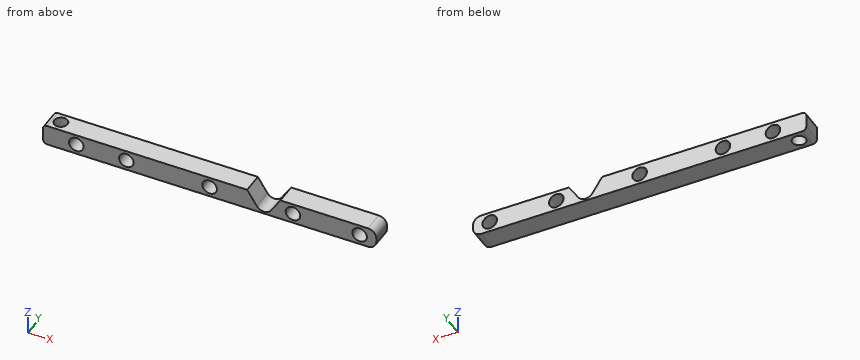
from build123d import *

# Parameters (mm, degrees)
SKETCH1_W           = 101.6
SKETCH1_H           = 6.35
BOSS_EXTRUDE1_DEPTH = 6.35
FILLET1_R           = 2.54
FILLET2_R           = 1.27
CUT_EXTRUDE1_REACH  = 53.294
SKETCH2_R           = 2.2225
CUT_EXTRUDE2_REACH  = 53.588
SKETCH3_R           = 2.032
CUT_EXTRUDE3_REACH  = 53.294


with BuildPart() as part:
    # Sketch1 → Boss-Extrude1 (new body)
    with BuildSketch(Plane(origin=(0, 0, 0), x_dir=(1, 0, 0), z_dir=(0, 1, 0))):
        Rectangle(SKETCH1_W, SKETCH1_H)
    extrude(amount=BOSS_EXTRUDE1_DEPTH)

    # Fillet1
    fillet1_edges = [part.edges().sort_by_distance(p)[0] for p in [
        (50.8, 3.175, 3.175),
        (50.8, 3.175, -3.175),
    ]]
    fillet(fillet1_edges, radius=FILLET1_R)

    # Fillet2
    fillet2_edges = [part.edges().sort_by_distance(p)[0] for p in [
        (-50.8, 3.175, 3.175),
        (-50.8, 3.175, -3.175),
    ]]
    fillet(fillet2_edges, radius=FILLET2_R)

    # Sketch2 → Cut-Extrude1 (cut, up to next)
    with BuildSketch(Plane(origin=(0, 6.35, 0), x_dir=(1, 0, 0), z_dir=(0, 1, 0)), mode=Mode.PRIVATE) as cut_extrude1_sk1:
        with Locations(Location((-40.64, 0, 0), (0, 0, 270))):
            Circle(SKETCH2_R)
    cut_extrude1_tool1 = extrude(cut_extrude1_sk1.sketch, amount=-CUT_EXTRUDE1_REACH, mode=Mode.PRIVATE) & part.part
    # Sketch2 → Cut-Extrude1 (cut, up to next)
    with BuildSketch(Plane(origin=(0, 6.35, 0), x_dir=(1, 0, 0), z_dir=(0, 1, 0)), mode=Mode.PRIVATE) as cut_extrude1_sk2:
        with Locations(Location((45.72, 0, 0), (0, 0, 270))):
            Circle(SKETCH2_R)
    cut_extrude1_tool2 = extrude(cut_extrude1_sk2.sketch, amount=-CUT_EXTRUDE1_REACH, mode=Mode.PRIVATE) & part.part
    # Sketch2 → Cut-Extrude1 (cut, up to next)
    with BuildSketch(Plane(origin=(0, 6.35, 0), x_dir=(1, 0, 0), z_dir=(0, 1, 0)), mode=Mode.PRIVATE) as cut_extrude1_sk3:
        with Locations(Location((25.4, 0, 0), (0, 0, 270))):
            Circle(SKETCH2_R)
    cut_extrude1_tool3 = extrude(cut_extrude1_sk3.sketch, amount=-CUT_EXTRUDE1_REACH, mode=Mode.PRIVATE) & part.part
    # Sketch2 → Cut-Extrude1 (cut, up to next)
    with BuildSketch(Plane(origin=(0, 6.35, 0), x_dir=(1, 0, 0), z_dir=(0, 1, 0)), mode=Mode.PRIVATE) as cut_extrude1_sk4:
        with Locations(Location((-25.4, 0, 0), (0, 0, 270))):
            Circle(SKETCH2_R)
    cut_extrude1_tool4 = extrude(cut_extrude1_sk4.sketch, amount=-CUT_EXTRUDE1_REACH, mode=Mode.PRIVATE) & part.part
    # Sketch2 → Cut-Extrude1 (cut, up to next)
    with BuildSketch(Plane(origin=(0, 6.35, 0), x_dir=(1, 0, 0), z_dir=(0, 1, 0)), mode=Mode.PRIVATE) as cut_extrude1_sk5:
        with Locations(Location((0, 0, 0), (0, 0, 270))):
            Circle(SKETCH2_R)
    cut_extrude1_tool5 = extrude(cut_extrude1_sk5.sketch, amount=-CUT_EXTRUDE1_REACH, mode=Mode.PRIVATE) & part.part
    add(cut_extrude1_tool1.solids().sort_by_distance((-40.64, 6.35, 0))[0], mode=Mode.SUBTRACT)
    add(cut_extrude1_tool2.solids().sort_by_distance((45.72, 6.35, 0))[0], mode=Mode.SUBTRACT)
    add(cut_extrude1_tool3.solids().sort_by_distance((25.4, 6.35, 0))[0], mode=Mode.SUBTRACT)
    add(cut_extrude1_tool4.solids().sort_by_distance((-25.4, 6.35, 0))[0], mode=Mode.SUBTRACT)
    add(cut_extrude1_tool5.solids().sort_by_distance((0, 6.35, 0))[0], mode=Mode.SUBTRACT)

    # Sketch3 → Cut-Extrude2 (cut, up to next)
    with BuildSketch(Plane.XY.offset(3.175), mode=Mode.PRIVATE) as cut_extrude2_sk1:
        with Locations((-46.99, 3.175)):
            Circle(SKETCH3_R)
    cut_extrude2_tool1 = extrude(cut_extrude2_sk1.sketch, amount=-CUT_EXTRUDE2_REACH, mode=Mode.PRIVATE) & part.part
    add(cut_extrude2_tool1.solids().sort_by_distance((-46.99, 3.175, 3.175))[0], mode=Mode.SUBTRACT)

    # Sketch4 → Cut-Extrude3 (cut, up to next)
    with BuildSketch(Plane(origin=(0, 6.35, 0), x_dir=(1, 0, 0), z_dir=(0, 1, 0)), mode=Mode.PRIVATE) as cut_extrude3_sk1:
        with BuildLine():
            Line((21.59, -3.175), (18.642458961, 1.379934338))
            ThreePointArc((18.642458961, 1.379934338), (16.51, 2.54), (14.377541039, 1.379934338))
            Line((14.377541039, 1.379934338), (11.43, -3.175))
            Line((11.43, -3.175), (21.59, -3.175))
        make_face()
    cut_extrude3_tool1 = extrude(cut_extrude3_sk1.sketch, amount=-CUT_EXTRUDE3_REACH, mode=Mode.PRIVATE) & part.part
    add(cut_extrude3_tool1.solids().sort_by_distance((16.51, 6.35, 0.914009))[0], mode=Mode.SUBTRACT)


solid = part.part
For this review, take the finished solid that the model builds, in its own axes (mm). Give positions to 0.01 mm unless a question says otherwise; leave off trailing zeros. Loops run counter-clockwise (first coordinate to the right, second up) from the corner with the lowest first, then second, coordinate; pieces in that order, holes last.
Item 1: For line 1 along Y through (x, z) = (-46.99, 0.25); line 2 along Z through (x, y) = (-1.5, 6) (3 decimals); line 3 along Z through (x, y) = (23.5, 0.75) (3 decimals), list the stretches that pass through material, from the lowest coordinate up.
Item 2: Insertion check: pin 1 (2 mm diameter, centred on x = 10, z = 0, fed in from -Y); pin 2 (3.5 mm diameter, centred on x = -40.64, z = 0, fed in from -Y); pin 3 (1.5 mm diameter, centred on y = 3.5, z = 2.5, fed in from +X). Each pin has a flat end and moves straight along its axis. Give the tip position at first contact, or say it passes through.
Item 3: Take a section at B-B, the plane y = 2. State the section outline as (x, z) points (1 decimal).
Calculated:
1. line 1: y = 0 to 1.14, 5.21 to 6.35
1. line 2: z = -3.175 to -1.64, 1.64 to 3.175
1. line 3: z = -3.175 to -1.153, 1.153 to 3.175
2. pin 1: stops at y = 0
2. pin 2: passes through
2. pin 3: stops at x = 50.54
3. outline: (-50.8, -1.9) arc R1.3 ccw to (-49.5, -3.2) - (-48.6, -3.2) - (-48.6, 3.2) - (-49.5, 3.2) arc R1.3 ccw to (-50.8, 1.9) - close; (-45.3, -3.2) - (48.3, -3.2) arc R2.5 ccw to (50.8, -0.6) - (50.8, 0.6) arc R2.5 ccw to (48.3, 3.2) - (21.6, 3.2) - (18.6, -1.4) arc R2.5 cw to (14.4, -1.4) - (11.4, 3.2) - (-45.3, 3.2) - close; hole circle Ø4.4 at (-40.6, 0); hole circle Ø4.4 at (-25.4, 0); hole circle Ø4.4 at (0, 0); hole circle Ø4.4 at (25.4, 0); hole circle Ø4.4 at (45.7, 0)
